Design review of the part built by this model. Coordinates are the model's own, in mm. Face numbers are marked on the shaded views. A direction names the side the tool comes from. Coordinates: 2 decimals unless noted, no trailing zeros. Loops run counter-clockwise (first coordinate to the right, second up) from the corner with the lowest first, then second, coordinate; pieces in that order, holes last. Notation, with made-up numbers: (33.5, 7) -> (45.5, 7) arc R21 cw to (45.5, 31) -> close; hole circle Ø8 at (-33.75, 54). An arc over 180 degrees is marked (long way). Answer in a Markdown table with one row per item.
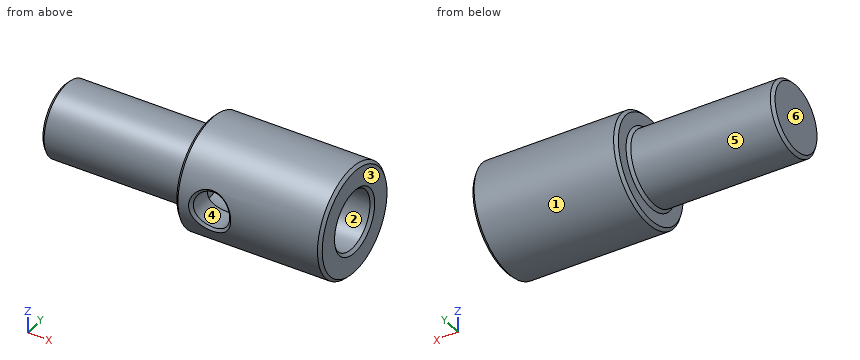
Autodesk Inventor part; units mm, degrees
ref_plane "YZ Plane" through (0, 0, 0) normal (1, 0, 0) x (0, 1, 0)
ref_plane "XZ Plane" through (0, 0, 0) normal (0, 1, 0) x (-1, 0, 0)
ref_plane "XY Plane" through (0, 0, 0) normal (0, 0, 1) x (1, 0, 0)
sketch "Sketch1" plane through (0, 0, 0) normal (1, 0, 0) x (0, 1, 0)
  circle A0 centre (0, 0) radius 3.175
  dimension "d0" = 6.35
extrude "Extrusion1" add sketch "Sketch1" along normal blind 12.7
sketch "Sketch2" plane through (12.7, 0, 0) normal (1, 0, 0) x (0, 0, -1)
  circle A0 centre (0, 0) radius 4.7625
  circle A1 centre (0, 0) radius 2.54
  dimension "d3" = 9.525
  dimension "d6" = 5.08
extrude "Extrusion2" add sketch "Sketch2" along normal blind 12.7
sketch "Sketch4" plane through (0, 0, 0) normal (0, 1, 0) x (-1, 0, 0)
  circle A0 centre (-15.7257, 0) radius 1.5875
  point P0 (0, 0)
  dimension "d7" = 3.175
extrude "Extrusion3" cut sketch "Sketch4" against normal up to next
chamfer "Chamfer1" distance 0.254 angle 45 6 edges at (0, -3.175, 0) (12.7, 0, 4.7625) (12.7, -3.175, 0) (17.2497, -4.7417, 0.4446) (25.4, 0, 4.7625) (25.4, 0, 2.54)
properties part number "Motor-Adapter"
(1) Take a section at B-B on x = 22.25. Give the boundary of the cut face in (y, z) (1 decimal), and give its area (3 significant figures).
Evaluation:
| item | result |
|---|---|
| outline | circle Ø9.5 at (0, 0); hole circle Ø5.1 at (0, 0) |
| area | 51.0 mm² |
(2) Tool access review of the marked faces 4, 5 and 6: name each direction out of +Z, -Z, +X, -X, +Y, -Y from which nothing blocks a thin tool from reaching the whole face with its end or side.
Evaluation:
| item | result |
|---|---|
| face 4 | -Y |
| face 5 | -X |
| face 6 | +Z, -Z, -X, +Y, -Y |
(3) To check wall thickness, follow probe 1 along Y at (x, z) = (22.5, 0); probe 2 along Z at (x, y) = (6, 1.25); probe 3 along X at (y, z) = (-2.5, 0). State the ranges of each line that lie inside material, in increasing order.
Evaluation:
| item | result |
|---|---|
| probe 1 | y = -4.76 to -2.54, 2.54 to 4.76 |
| probe 2 | z = -2.92 to 2.92 |
| probe 3 | x = 0 to 12.7 |
(4) Draft analysis for pull direction Y (two halves, no side actions). For the marked faces 1, 2 and 3, state which applies: pulls with the +Y half, pulls with the -Y half, needs draft (parallel to the pull), parting line crosses it, or undercut.
Evaluation:
| item | result |
|---|---|
| face 1 | parting line crosses it |
| face 2 | undercut |
| face 3 | needs draft |
(5) For pin 1 (4 mm diameter, centred on y = -0.5, z = 0.5, fed in from +X); pin 2 (1.5 mm diameter, centred on x = 13, z = 2, fed in from +Y); pin 3 (1.5 mm diameter, centred on x = 5, z = -2.5, fed in from +Y), all flat-tipped, find the tip position at first contact; note any pin that passes through.
Evaluation:
| item | result |
|---|---|
| pin 1 | stops at x = 25.31 |
| pin 2 | stops at y = 4.6 |
| pin 3 | stops at y = 2.65 |
